Model file for the job. Use its own axes, mm. Round coordinates to 2 decimals unless told otherwise and drop trailing zeros. Order: outer loops, then holes, each group sorted by start corner. A loop starts at its lowest first (then second) coordinate and runs counter-clockwise, first axis right, second up. Notation, with made-up numbers: (78.5, 3.25) -> (128.5, 3.25) arc R23 cw to (128.5, 41.25) -> close; hole circle Ø6 at (-21, 85). An arc over 180 degrees is marked (long way). Use CSV: the item, a comma, the result in double quotes.
```python
from build123d import *

# Parameters (mm, degrees)
ESTRUSIONE_ESTRUSIONE1_DEPTH = 5
TAGLIO_ESTRUSIONE1_DEPTH     = 10
RIPETIZIONECIRCOLARE1_COUNT  = 3


with BuildPart() as part:
    # Schizzo1 → Estrusione-Estrusione1 (new, symmetric)
    with BuildSketch(Plane(origin=(0, 0, 0), x_dir=(1, 0, 0), z_dir=(0, 1, 0))):
        Polygon((-24, -13.856406461), (0, 27.712812921), (24, -13.856406461), align=None)
    extrude(amount=ESTRUSIONE_ESTRUSIONE1_DEPTH, both=True)

    # Schizzo2 → Taglio-Estrusione1 (cut)
    with BuildSketch(Plane(origin=(0, 5, 0), x_dir=(1, 0, 0), z_dir=(0, 1, 0))):
        Polygon((14, -13.856406461), (19, -5.196152423), (24, -13.856406461), align=None)
    taglio_estrusione1 = extrude(amount=-TAGLIO_ESTRUSIONE1_DEPTH, mode=Mode.SUBTRACT)

    # RipetizioneCircolare1: Taglio-Estrusione1 ×3 about axis
    ripetizionecircolare1_axis = Axis((0, 0, 0), (0, 1, 0))
    for i in range(1, RIPETIZIONECIRCOLARE1_COUNT):
        add(taglio_estrusione1.rotate(ripetizionecircolare1_axis, i * 360 / RIPETIZIONECIRCOLARE1_COUNT), mode=Mode.SUBTRACT)


solid = part.part
```
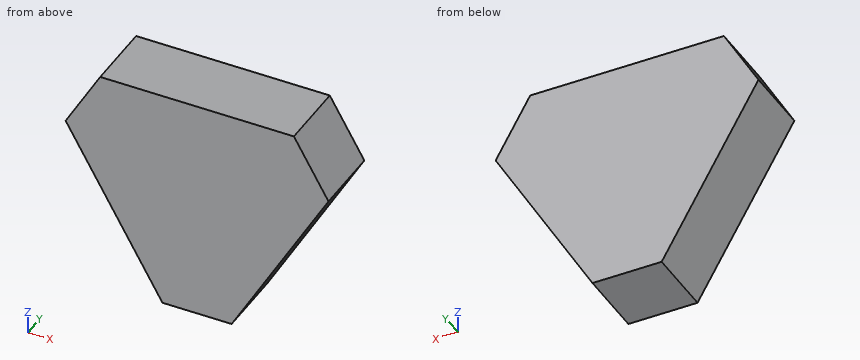
Q1. Cut at A-A (y = -2). Give the cut face in (x, z).
From the geometry:
outline,"(-19, 5.2) -> (-5, -19.05) -> (5, -19.05) -> (19, 5.2) -> (14, 13.86) -> (-14, 13.86) -> close"
Q2. Probe line 1 along X through (y, z) = (-1.25, 12); line 2 along X through (y, z) = (-2.75, 12.5); line 3 along Z through (x, y) = (-10, 4.5). List the from-to ranges inside material, lowest first.
From the geometry:
line 1,"x = -15.07 to 15.07"
line 2,"x = -14.78 to 14.78"
line 3,"z = -10.39 to 13.86"
Q3. Pin check, flat tips, straight feed: pin 1 (1 mm diameter, centred on x = -7, y = 2.5, fed in from -Z); pin 2 (2 mm diameter, centred on y = 2.5, z = -5, fed in from +X); pin 3 (1.5 mm diameter, centred on x = -10, y = -1.5, fed in from -Z). Stop position of each tip, or through.
From the geometry:
pin 1,"stops at z = -16.45"
pin 2,"stops at x = 13.69"
pin 3,"stops at z = -11.69"
Q4. Cut at C-C (z = -4.5). Give the cut face in (x, y), plus the area to 3 significant figures.
From the geometry:
outline,"(-13.4, -5) -> (13.4, -5) -> (13.4, 5) -> (-13.4, 5) -> close"
area,"268 mm²"
Q5. Cut at B-B (x = 11). Give the cut face in (y, z).
From the geometry:
outline,"(-5, -8.66) -> (5, -8.66) -> (5, 13.86) -> (-5, 13.86) -> close"
